```python
from build123d import *

# Parameters (mm, degrees)
HOLE1_D           = 6.4389
HOLE1_DEPTH       = 40.4876
HOLE1_CSINK_D     = 6.9469
HOLE1_CSINK_ANGLE = 90
SKETCH5_W         = 3.175
SKETCH5_H         = 5.08


with BuildPart() as part:
    # Sketch1 → Revolve1 (revolve)
    with BuildSketch(Plane.XY):
        with BuildLine():
            Line((0, 0), (0, 7.09803))
            Line((0, 7.09803), (0.83947, 7.9375))
            Line((0.83947, 7.9375), (6.681592328, 7.9375))
            Line((6.681592328, 7.9375), (7.520171502, 7.096504435))
            ThreePointArc((7.520171502, 7.096504435), (7.804772216, 6.905895804), (8.1407, 6.83895))
            Line((8.1407, 6.83895), (9.4361, 6.83895))
            ThreePointArc((9.4361, 6.83895), (10.055737672, 7.095612328), (10.3124, 7.71525))
            Line((10.3124, 7.71525), (10.3124, 7.90575))
            Line((10.3124, 7.90575), (12.7, 7.90575))
            Line((12.7, 7.90575), (12.7, 0))
            Line((12.7, 0), (0, 0))
        make_face()
    revolve(axis=Axis((12.7, 0, 0), (-1, 0, 0)))

    # Sketch2 → Revolve2 (revolve)
    with BuildSketch(Plane.XY):
        Polygon((12.7, 0), (12.7, 10.19175), (13.462, 10.95375), (34.0741, 10.95375), (34.0741, 8.90905), (34.8361, 8.90905), (35.5981, 9.67105), (39.7256, 9.67105), (40.4876, 8.90905), (40.4876, 0), align=None)
    revolve(axis=Axis((40.4876, 0, 0), (-1, 0, 0)))

    # Hole1
    with Locations(Plane.ZY):
        with Locations((0, 0)):
            CounterSinkHole(HOLE1_D / 2, HOLE1_CSINK_D / 2, depth=HOLE1_DEPTH, counter_sink_angle=HOLE1_CSINK_ANGLE)

    # Sketch5 → Cut-Revolve1 (revolve, cut)
    with BuildSketch(Plane.XY):
        with Locations((32.4866, 12.79525)):
            Rectangle(SKETCH5_W, SKETCH5_H)
    revolve(axis=Axis((34.0741, 0, 0), (-1, 0, 0)), mode=Mode.SUBTRACT)

    # Sketch6 → Cut-Revolve2 (revolve, cut)
    with BuildSketch(Plane(origin=(0, 0, 0), x_dir=(1, 0, 0), z_dir=(0, 1, 0))):
        Polygon((24.6126, 0), (27.7876, 0), (27.7876, -3.137518166), (29.253831834, -4.60375), (29.452075925, -10.95375), (24.6126, -10.95375), align=None)
    revolve(axis=Axis((24.6126, 0, 10.95375), (0, 0, -1)), mode=Mode.SUBTRACT)

    # Sketch7 → Revolve3 (revolve)
    with BuildSketch(Plane.XY):
        with BuildLine():
            Line((34.0741, 8.65505), (34.8361, 8.65505))
            Line((34.8361, 8.65505), (34.8361, 8.90905))
            Line((34.8361, 8.90905), (34.4551, 8.90905))
            Line((34.4551, 8.90905), (34.196587194, 9.167562806))
            ThreePointArc((34.196587194, 9.167562806), (34.159389755, 9.257365367), (34.196587194, 9.347167928))
            Line((34.196587194, 9.347167928), (35.02050107, 10.171081804))
            Line((35.02050107, 10.171081804), (35.02050107, 10.25525))
            Line((35.02050107, 10.25525), (34.81730107, 10.25525))
            Line((34.81730107, 10.25525), (34.0741, 9.51204893))
            Line((34.0741, 9.51204893), (34.0741, 8.65505))
        make_face()
    revolve(axis=Axis((34.8361, 0, 0), (-1, 0, 0)))


solid = part.part
```
Here's how the part is built. I have some questions about the finished solid (model axes, mm). A direction names the side the tool comes from. Round coordinates to 2 decimals unless told otherwise and drop trailing zeros. Loops run counter-clockwise (first coordinate to the right, second up) from the corner with the lowest first, then second, coordinate; pieces in that order, holes last. Notation, with made-up numbers: (-36.5, -38.75) -> (-30.5, -38.75) arc R17 cw to (-30.5, -32.75) -> close; hole circle Ø8 at (71.5, -4.5). An arc over 180 degrees is marked (long way). Answer as CSV lines item,"result". Start each with the question number.
1. Imagine slicing it at C-C on x = 33.5. Write out the boundary of the cut face in (y, z).
2. If we mould it in two halves opening along X, with no side actions, what happens to faces 5 (the face through (34.648, 8.498, -2.676)), 6 (the face through (40.488, 4, 0)), 7 (the face through (37.691, 9.224, -2.905))? For each: pulls with the +X half, pulls with the -X half, needs draft (parallel to the pull), parting line crosses it, or undercut.
3. I need wall thicknesses on probe 1 along Z at (x, y) = (12, 0); probe 2 along Y at (x, z) = (26.5, 0). Which ranges of each line are inside material? Lowest first, please. Write a range as from..to.
4. Imagine slicing it at A-A on x = 3.5. Write out the boundary of the cut face in (y, z) (1 decimal).
5. Imagine slicing it at B-B on y = 0. State how many separate pieces and enclosed holes the cut face has, plus the area to 3 significant figures.
6. I'm going to push flat-ended pins straight in: P1, Ø2, axis at x = 32.5, z = -5, coming from the -Y side; P2, Ø6, axis at x = 14, y = 8.5, coming from the +Z side; P3, Ø1.5, axis at y = -6.5, z = -8, coming from the -X side. Where does each tip first touch, or does it pass through?
7. For faces 1 (the face through (32.509, -2.223, 10.011)), 2 (the face through (24.672, -3.174, 2.143)), 3 (the face through (11.523, -6.274, 4.811)), 4 (the face through (3.8, -1.72, 7.75)), which set-ups out of +Z, -Z, +X, -X, +Y, -Y let a thin tool reach every point of the face, with its end or its side?
Solution:
1,outline,"circle Ø20.51 at (0, 0); hole circle Ø6.44 at (0, 0)"
2,face 5,"undercut"
2,face 6,"pulls with the +X half"
2,face 7,"needs draft"
3,probe 1,"-7.91..-3.22, 3.22..7.91"
3,probe 2,"-10.95..-3.22, 3.22..10.95"
4,outline,"circle Ø15.9 at (0, 0); hole circle Ø6.4 at (0, 0)"
5,separate pieces,"3"
5,enclosed holes,"0"
5,area,"448 mm²"
6,P1,"y = -9.44"
6,P2,"z = 9.47"
6,P3,"x = 12.7"
7,face 1,"+X"
7,face 2,"+Z"
7,face 3,"none"
7,face 4,"-X"
